from build123d import *

# Parameters (mm, degrees)
SKETCH1_W               = 325.9836
SKETCH1_H               = 197.27926
BOSS_EXTRUDE1_DEPTH     = 3.175
F_1_4_CLEARANCE_HOLE1_D = 7.14248
SKETCH4_W               = 3.175
SKETCH4_H               = 152.4
SKETCH4_W_2             = 254
SKETCH4_H_2             = 3.175
CUT_EXTRUDE1_DEPTH      = 191.541817192


with BuildPart() as part:
    # Sketch1 → Boss-Extrude1 (new body)
    with BuildSketch(Plane(origin=(0, 0, 0), x_dir=(1, 0, 0), z_dir=(0, 1, 0))):
        Rectangle(SKETCH1_W, SKETCH1_H)
    extrude(amount=BOSS_EXTRUDE1_DEPTH)

    # 1/4 Clearance Hole1 (through all)
    with Locations(Plane(origin=(0, 3.175, 0), x_dir=(1, 0, 0), z_dir=(0, 1, 0))):
        with Locations((-150.2918, 85.93963), (150.2918, 85.93963), (150.2918, -85.93963), (-150.2918, -85.93963)):
            Hole(F_1_4_CLEARANCE_HOLE1_D / 2)

    # Sketch4 → Cut-Extrude1 (cut, through all)
    with BuildSketch(Plane(origin=(0, 3.175, 0), x_dir=(1, 0, 0), z_dir=(0, 1, 0))):
        with Locations((-150.2918, 0)):
            Rectangle(SKETCH4_W, SKETCH4_H)
        with Locations((150.2918, 0)):
            Rectangle(SKETCH4_W, SKETCH4_H)
        with Locations((0, 85.93963)):
            Rectangle(SKETCH4_W_2, SKETCH4_H_2)
        with Locations((0, -85.93963)):
            Rectangle(SKETCH4_W_2, SKETCH4_H_2)
    extrude(amount=-CUT_EXTRUDE1_DEPTH, mode=Mode.SUBTRACT)


solid = part.part
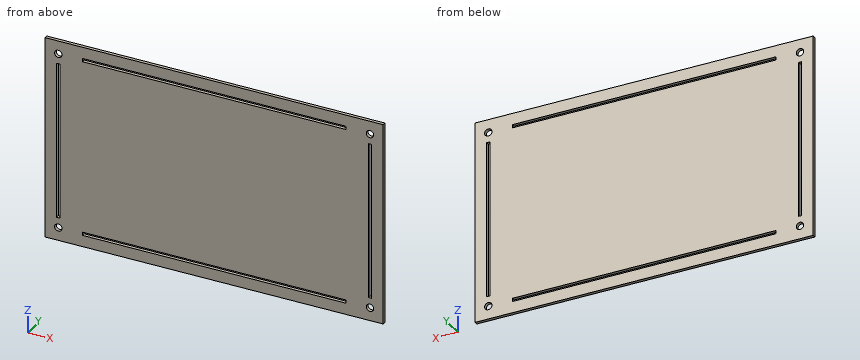
Can you work these out from the model? Positions are in its coordinate system, mm. Give positions to 0.01 mm unless a question says otherwise; leave off trailing zeros. Order: outer loops, then holes, each group sorted by start corner. A loop starts at its lowest first (then second) coordinate and runs counter-clockwise, first axis right, second up. Notation, with made-up numbers: M 5.5,-24.75 L 43.5,-24.75 A16 cw 43.5,-20.75 Z; hole C -6,51 d6. An arc over 180 degrees is marked long. Use a Markdown table: item, result. Add a question column.
Item 1: Will this pin go through, and if not, where does the flat tip stop? pin 1 (5.5 mm diameter, centred on x = 150.29, z = -85.94, fed in from +Y).
Item 2: Suppose I cut it at A-A (z = 45.5). List the corners of the cut face in (x, y) for me (3 decimals), then the cut area to 3 significant figures.
Item 3: If I drill on L1, parallel to Z at x = 74, y = 0.35; L2, parallel to X at y = 1.7, z = -86; L3, parallel to X at y = 1.8, z = -26.5, over which ranges is the centre line in solid material (lowest first)? Write a range as [from, to].
Item 4: Suppose I cut it at B-B (x = -91). List the corners of the cut face in (y, z) for me (3 decimals), then the cut area to 3 significant figures.
Item 5: Suppose I cut it at C-C (y = 2.5). Count the separate pieces of the cut face and the enclosed holes in it, then the cut area to 3 significant figures.
Answer sheet:
| question | item | result |
|---|---|---|
| 1 | pin 1 | passes through |
| 2 | outline | M -162.992,0 L -151.879,0 L -151.879,3.175 L -162.992,3.175 Z; M -148.704,0 L 148.704,0 L 148.704,3.175 L -148.704,3.175 Z; M 151.879,0 L 162.992,0 L 162.992,3.175 L 151.879,3.175 Z |
| 2 | area | 1,010 mm² |
| 3 | L1 | z = [-98.64, -87.53], [-84.35, 84.35], [87.53, 98.64] |
| 3 | L2 | x = [-162.99, -153.86], [-146.72, -127], [127, 146.72], [153.86, 162.99] |
| 3 | L3 | x = [-162.99, -151.88], [-148.7, 148.7], [151.88, 162.99] |
| 4 | outline | M 0,-98.64 L 3.175,-98.64 L 3.175,-87.527 L 0,-87.527 Z; M 0,-84.352 L 3.175,-84.352 L 3.175,84.352 L 0,84.352 Z; M 0,87.527 L 3.175,87.527 L 3.175,98.64 L 0,98.64 Z |
| 4 | area | 606 mm² |
| 5 | separate pieces | 1 |
| 5 | enclosed holes | 8 |
| 5 | area | 61,600 mm² |
